```python
from build123d import *

# Parameters (mm, degrees)
SKETCH1_W           = 30
SKETCH1_H           = 30
BOSS_EXTRUDE1_DEPTH = 16
SKETCH2_R           = 2.5
CUT_EXTRUDE1_DEPTH  = 46.343136195
SKETCH3_R           = 4
CUT_EXTRUDE2_DEPTH  = 46.343136195
FILLET1_R           = 8
FILLET2_R           = 3


with BuildPart() as part:
    # Sketch1 → Boss-Extrude1 (new body)
    with BuildSketch(Plane.XY):
        with Locations((15, 15)):
            Rectangle(SKETCH1_W, SKETCH1_H)
    extrude(amount=BOSS_EXTRUDE1_DEPTH)

    # Sketch2 → Cut-Extrude1 (cut, through all)
    with BuildSketch(Plane(origin=(0, 0, 0), x_dir=(-1, 0, 0), z_dir=(0, 0, -1))):
        with Locations((-15, 15)):
            Circle(SKETCH2_R)
    extrude(amount=-CUT_EXTRUDE1_DEPTH, mode=Mode.SUBTRACT)

    # Sketch3 → Cut-Extrude2 (cut, through all)
    with BuildSketch(Plane(origin=(0, 30, 0), x_dir=(1, 0, 0), z_dir=(0, 1, 0))):
        with Locations(Location((15, -8, 0), (0, 0, 270))):
            Circle(SKETCH3_R)
    extrude(amount=-CUT_EXTRUDE2_DEPTH, mode=Mode.SUBTRACT)

    # Fillet1
    fillet1_edges = [part.edges().sort_by_distance(p)[0] for p in [
        (30, 15, 0),
        (30, 15, 16),
        (0, 15, 0),
        (0, 15, 16),
    ]]
    fillet(fillet1_edges, radius=FILLET1_R - 0.0001)  # a hair under: the kernel refuses the full size

    # Fillet2
    fillet2_edges = [part.edges().sort_by_distance(p)[0] for p in [
        (15, 30, 0),
        (15, 30, 16),
        (2.343116461, 30, 13.656883539),
        (2.343116461, 30, 2.343116461),
        (27.656883539, 30, 13.656883539),
        (27.656883539, 30, 2.343116461),
        (15, 0, 0),
        (15, 0, 16),
        (2.343116461, 0, 13.656883539),
        (2.343116461, 0, 2.343116461),
        (27.656883539, 0, 13.656883539),
        (27.656883539, 0, 2.343116461),
    ]]
    fillet(fillet2_edges, radius=FILLET2_R)


solid = part.part
```
Work out the finished part from the listing and answer in its coordinate system (mm). Give positions to 0.01 mm unless a question says otherwise; leave off trailing zeros. Loops run counter-clockwise (first coordinate to the right, second up) from the corner with the lowest first, then second, coordinate; pieces in that order, holes last. Notation, with made-up numbers: M 13,77.25 L 50,77.25 A35 ccw 50,113.25 Z; hole C -26,74.25 d4. An arc over 180 degrees is marked long. One line per item, written item: value. Start each with the question number.
1. Each of these flat-tipped pins is pushed along its axis until it touches: P1, Ø1.5, axis at y = 17.5, z = 7, coming from the +X side; P2, Ø2, axis at y = 17.5, z = 11.5, coming from the -X side. Where does it stop, or does it pass through?
2. Find section B-B (x = 15). Give the vertices of the cut face in (y, z).
3. Find section C-C (x = 21). Give the vertices of the cut face in (y, z), and give its area (3 significant figures).
4. Determine the mould class of faces 1 (the face through (15.1, 0.86, 0.9)), 2 (the face through (14.9, 0.86, 15.1)), 3 (the face through (17.5, 0, 4.6)), 4 (the face through (18.966, 15.21, 7.479)) for opening direction Z: released by +Z, released by -Z, zero draft, split by the parting line, or undercut.
5. Find the intervals of material crossed by probe 1 along Y at (x, z) = (15, 12.8); probe 2 along Z at (x, y) = (15.25, 12); probe 3 along X at (y, z) = (22.5, 8), in increasing order.
Reported:
1. P1: stops at x = 30
1. P2: stops at x = 0.4
2. outline: M 0,3 A3 ccw 3,0 L 12.5,0 L 12.5,4 L 0,4 Z; M 0,12 L 12.5,12 L 12.5,16 L 3,16 A3 ccw 0,13 Z; M 17.5,0 L 27,0 A3 ccw 30,3 L 30,4 L 17.5,4 Z; M 17.5,12 L 30,12 L 30,13 A3 ccw 27,16 L 17.5,16 Z
3. outline: M 0,3 A3 ccw 3,0 L 27,0 A3 ccw 30,3 L 30,13 A3 ccw 27,16 L 3,16 A3 ccw 0,13 Z
3. area: 472 mm²
4. face 1: released by -Z
4. face 2: released by +Z
4. face 3: zero draft
4. face 4: undercut
5. probe 1: y = 0 to 12.5, 17.5 to 30
5. probe 2: z = 0 to 4.01, 11.99 to 16
5. probe 3: x = 0 to 11, 19 to 30
